```python
from build123d import *

# Parameters (mm, degrees)
CUT_EXTRUDE_578_DEPTH      = 70.85
PATTERN_CIRCULAR_632_COUNT = 5
SKETCH_7_R                 = 51
EXTRUDE_1_DEPTH            = 10
CUT_EXTRUDE_START          = -1.5
SKETCH_8_R                 = 51
SKETCH_8_R_2               = 45
CUT_EXTRUDE_1_DEPTH        = 1.5
SKETCH_10_R                = 2.75
CUT_EXTRUDE_5_DEPTH        = 8
CUT_EXTRUDE_6_REACH        = 89.761
SKETCH_11_W                = 20
SKETCH_11_H                = 4
SKETCH_11_W_2              = 5.5
SKETCH_11_H_2              = 10.5


with BuildPart() as part:
    # Эскиз2 → Revolve 375 (revolve)
    with BuildSketch(Plane.XY, mode=Mode.PRIVATE) as revolve_375_sk:
        with BuildLine():
            Line((0, 0), (-49.5, 0))
            Line((-49.5, 0), (-49.5, -40))
            Line((-49.5, -40), (-47.5, -40))
            Line((-47.5, -40), (-47.5, -5.5))
            ThreePointArc((-47.5, -5.5), (-46.621320344, -3.378679656), (-44.5, -2.5))
            Line((-44.5, -2.5), (0, -2.5))
            Line((0, -2.5), (0, 0))
        make_face()
    revolve(revolve_375_sk.sketch.rotate(Axis((0, 0, 0), (0, 1, 0)), 270), axis=Axis((0, 0, 0), (0, 1, 0)))

    # Эскиз4 → Cut-Extrude 578 (cut, symmetric)
    with BuildSketch(Plane.XY):
        Polygon((-8, -7), (8, -7), (0, -37), align=None)
    cut_extrude_578 = extrude(amount=CUT_EXTRUDE_578_DEPTH, both=True, mode=Mode.SUBTRACT)

    # Pattern Circular 632: Cut-Extrude 578 ×5 about axis
    pattern_circular_632_axis = Axis((0, 0, 0), (0, 1, 0))
    for i in range(1, PATTERN_CIRCULAR_632_COUNT):
        add(cut_extrude_578.rotate(pattern_circular_632_axis, i * 360 / PATTERN_CIRCULAR_632_COUNT), mode=Mode.SUBTRACT)

    # Эскиз7 → Бобышка-Вытянуть1 (add)
    with BuildSketch(Plane(origin=(0, 0, 0), x_dir=(1, 0, 0), z_dir=(0, 1, 0))):
        with Locations(Location((0, 0, 0), (0, 0, 270))):
            Circle(SKETCH_7_R)
    extrude(amount=EXTRUDE_1_DEPTH)

    # Эскиз8 → Вырез-Вытянуть1 (cut)
    with BuildSketch(Plane(origin=(0, 10, 0), x_dir=(1, 0, 0), z_dir=(0, 1, 0)).offset(CUT_EXTRUDE_START)):
        with Locations(Location((0, 0, 0), (0, 0, 270))):
            Circle(SKETCH_8_R)
        with Locations(Location((0, 0, 0), (0, 0, 270))):
            Circle(SKETCH_8_R_2, mode=Mode.SUBTRACT)
    extrude(amount=CUT_EXTRUDE_1_DEPTH, mode=Mode.SUBTRACT)

    # Эскиз10 → Вырез-Вытянуть5 (cut)
    with BuildSketch(Plane(origin=(0, 10, 0), x_dir=(1, 0, 0), z_dir=(0, 1, 0))):
        with Locations(Location((0, -30, 0), (0, 0, 270))):
            Circle(SKETCH_10_R)
        with Locations(Location((-25.980762114, 15, 0), (0, 0, 270))):
            Circle(SKETCH_10_R)
        with Locations(Location((25.980762114, 15, 0), (0, 0, 270))):
            Circle(SKETCH_10_R)
    extrude(amount=-CUT_EXTRUDE_5_DEPTH, mode=Mode.SUBTRACT)

    # Эскиз11 → Вырез-Вытянуть6 (cut, up to next)
    with BuildSketch(Plane(origin=(0, 10, 0), x_dir=(1, 0, 0), z_dir=(0, 1, 0)), mode=Mode.PRIVATE) as cut_extrude_6_sk1:
        with Locations((4, 4)):
            Rectangle(SKETCH_11_W, SKETCH_11_H)
    cut_extrude_6_tool1 = extrude(cut_extrude_6_sk1.sketch, amount=-CUT_EXTRUDE_6_REACH, mode=Mode.PRIVATE) & part.part
    # Эскиз11 → Вырез-Вытянуть6 (cut, up to next)
    with BuildSketch(Plane(origin=(0, 10, 0), x_dir=(1, 0, 0), z_dir=(0, 1, 0)), mode=Mode.PRIVATE) as cut_extrude_6_sk2:
        with Locations((-23, 0)):
            Rectangle(SKETCH_11_W_2, SKETCH_11_H_2)
    cut_extrude_6_tool2 = extrude(cut_extrude_6_sk2.sketch, amount=-CUT_EXTRUDE_6_REACH, mode=Mode.PRIVATE) & part.part
    add(cut_extrude_6_tool1.solids().sort_by_distance((4, 10, -4))[0], mode=Mode.SUBTRACT)
    add(cut_extrude_6_tool2.solids().sort_by_distance((-23, 10, 0))[0], mode=Mode.SUBTRACT)


solid = part.part
```
Geometry: final body of the model. Coordinates: model frame, mm. A direction names the side the tool comes from. Round coordinates to 2 decimals unless told otherwise and drop trailing zeros. Loops run counter-clockwise (first coordinate to the right, second up) from the corner with the lowest first, then second, coordinate; pieces in that order, holes last. Notation, with made-up numbers: (20.25, 69.25) -> (68.25, 69.25) arc R22 ccw to (68.25, 83.25) -> close; hole circle Ø4 at (51.5, 13.5). An arc over 180 degrees is marked (long way). Use one line per item in the form item = value. Start each with the question number.
1) Section B-B on y = -35. Give the number of separate pieces and of enclosed holes in the cut face, then the cut area to 3 significant figures.
2) Line query: L1, parallel to X at y = -18.5, z = 0; L2, parallel to X at y = 4.5, z = -15; L3, parallel to Y at x = 3, z = -12. Output: solid intervals per line, ascending.
3) First-contact query: P1, Ø3.5, axis at x = -25.98, z = -15, coming from the +Y side; P2, Ø5, axis at y = 5, z = -1, coming from the -X side; P3, Ø2, axis at x = -26, y = -20, coming from the -Z side; P4, Ø1, axis at x = 5.5, z = -4, coming from the +Y side. Flat tips, straight axial feed; report the tip coordinate or a pass-through.
4) Access query for faces 1 (the cylindrical face through (-14.868, -20.28, -47.214)), 2 (the flat face through (26, 2, -15)), 3 (the flat face through (-6, 4, -4)). Directions: +Z, -Z, +X, -X, +Y, -Y. A direction counts if a zero-diameter tool reaches every point of the face in a straight line with its end or side. Return the directions, or none.
5) Draft query along Y for faces 4 (the flat face through (28, -7, 39)), 5 (the flat face through (-44, -40, 19)), 6 (the cylindrical face through (0.121, 6.056, 27.253)), 7 (the flat face through (-46, -7, 15)). Return one class per face: released by +Y, released by -Y, zero draft, split by the parting line, or undercut.
6) Section A-A on z = 0. Output: boundary loops of the cut face in (x, y).
Response:
q1.separate_pieces = 10
q1.enclosed_holes = 0
q1.area = 588 mm^2
q2.L1 = -49.5 to -47.5, 47.5 to 49.5
q2.L2 = -48.74 to -28.73, -23.23 to 23.23, 28.73 to 48.74
q2.L3 = -2.5 to 10
q3.P1 = 2
q3.P2 = -51
q3.P3 = -42.72
q3.P4 = through
q4.face_1 = -Y
q4.face_2 = +Y
q4.face_3 = +Y, -Y
q5.face_4 = undercut
q5.face_5 = released by -Y
q5.face_6 = zero draft
q5.face_7 = undercut
q6.outline = (-51, 0) -> (-49.5, 0) -> (-49.5, -40) -> (-47.5, -40) -> (-47.5, -5.5) arc R3 cw to (-44.5, -2.5) -> (-25.75, -2.5) -> (-25.75, 10) -> (-45, 10) -> (-45, 8.5) -> (-51, 8.5) -> close; (-20.25, -2.5) -> (44.5, -2.5) arc R3 cw to (47.5, -5.5) -> (47.5, -40) -> (49.5, -40) -> (49.5, 0) -> (51, 0) -> (51, 8.5) -> (45, 8.5) -> (45, 10) -> (-20.25, 10) -> close
